Source: CAD feature listing. Evaluate the final solid. Frame: model axes, mm. Face numbers are marked on the shaded views. A direction names the side the tool comes from. Round coordinates to 2 decimals unless told otherwise and drop trailing zeros. Loops run counter-clockwise (first coordinate to the right, second up) from the corner with the lowest first, then second, coordinate; pieces in that order, holes last. Notation, with made-up numbers: (9.5, 0) -> (20.5, 0) arc R21 ccw to (20.5, 39) -> close; hole circle Ø6 at (64, 86.5). An arc over 180 degrees is marked (long way). Put each result on its own line as item: value. Start each with the question number.
1. Cut plane A-A (z = 26). Return the cut outline in (x, y), then the cut area to 3 significant figures.
2. Contact query for flat-ended pins moving along their axis: pin 1 (1.6 mm diameter, centred on x = -38.37, z = 26.15, fed in from +Y); pin 2 (1.5 mm diameter, centred on y = -3.5, z = 33.5, fed in from -X); pin 3 (2 mm diameter, centred on y = -3, z = 30.5, fed in from -X). Output: stop coordinate, or through.
3. Cut plane D-D (x = -34.75). Return the cut outline in (y, z), then the cut area to 3 significant figures.
4. Draft query along Z for the marked faces 1, 2 and 3. Return one class per face: pulls with the +Z half, pulls with the -Z half, needs draft (parallel to the pull), parting line crosses it, or undercut.
5. Cut plane B-B (y = -3.5). State how many separate pieces and enclosed holes the cut face has, then the cut area to 3 significant figures.
6. Material intervals for L1, parallel to Z at x = -30.75, y = -2.5; L2, parallel to Z at x = -38.25, y = -0.5; L3, parallel to X at y = -3.6, z = 28.25, sorted ascending.
7. Set-up query: the marked faces 4, 5 and 6. Return all of +Z, -Z, +X, -X, +Y, -Y with unobstructed straight access to the full face (end or side cutting, diameter ignored); none if empty.
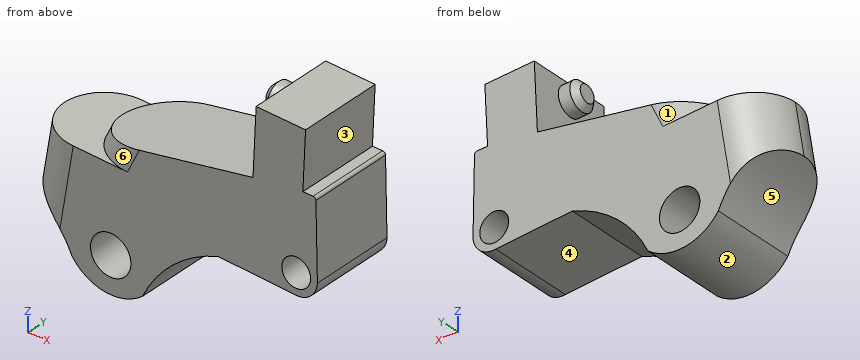
```python
from build123d import *

# Parameters (mm, degrees)
F1_DEPTH = 3.81
F2_D     = 1.778
F3_D     = 1.27
F4_R     = 1.90499
F5_DEPTH = 2.921
F6_R     = 0.636089801
F7_DEPTH = 0.762
F8_SIZE  = 0.254
F9_R     = 0.127


# Not quite as in the source:
# - a fillet or chamfer is up to 0.001 mm smaller than in the source, because OpenCascade refuses the exact size
# - a feature names something its author has since deleted; it is built from what else it names


with BuildPart() as f1:
    # F0 (on Front) → F1 (new body)
    with BuildSketch(Plane.XZ):
        with BuildLine():
            Line((-39.4140869416, 30.484917322), (-39.6941413215, 29.9037330352))
            Line((-39.6941413215, 29.9037330352), (-41.9326054958, 30.025163579))
            Line((-41.9326054958, 30.025163579), (-42.315851897, 27.6998355985))
            ThreePointArc((-42.315851897, 27.6998355985), (-40.9839410359, 26.7856748681), (-40.0724932551, 25.4519060254))
            ThreePointArc((-40.0724932551, 25.4519060254), (-38.6103077884, 24.5752589314), (-36.9695164263, 25.0381845981))
            ThreePointArc((-36.9695164263, 25.0381845981), (-35.6119860231, 26.8367061404), (-33.6415685093, 27.929877378))
            Line((-33.6415685093, 27.929877378), (-30.2701074994, 27.6978733483))
            ThreePointArc((-30.2701074994, 27.6978733483), (-29.5830798604, 27.8997588647), (-29.2723267028, 28.5448923498))
            Line((-29.2723267028, 28.5448923498), (-29.339633882, 31.9740138948))
            Line((-29.339633882, 31.9740138948), (-29.925275594, 31.9827347994))
            Line((-29.925275594, 31.9827347994), (-29.9314986914, 31.6059216857))
            Line((-29.9314986914, 31.6059216857), (-32.1076634707, 31.7085161805))
            Line((-32.1076634707, 31.7085161805), (-39.4140869416, 30.484917322))
        make_face()
    extrude(amount=F1_DEPTH)

    # F2 (through all)
    with Locations(Plane(origin=(0, 0, 0), x_dir=(1, 0, 0), z_dir=(0, 1, 0))):
        with Locations((-38.3695736527, -26.1525325477)):
            Hole(F2_D / 2)

    # F3 (through all)
    with Locations(Plane(origin=(0, 0, 0), x_dir=(1, 0, 0), z_dir=(0, 1, 0))):
        with Locations((-30.2061401308, -28.6094471812)):
            Hole(F3_D / 2)

    # F4 (radius 1.905 in the source; OpenCascade refuses exactly that, so slightly less here)
    f4_edges = [f1.edges().sort_by_distance(p)[0] for p in [
        (-42.124229, -3.81, 28.8625),
        (-42.124229, 0, 28.8625),
        (-39.554114, -3.81, 30.194325),
        (-39.554114, 0, 30.194325),
    ]]
    fillet(f4_edges, radius=F4_R)

    # F5 (add): a face of the model
    f5_faces = [f1.faces().sort_by_distance(p)[0] for p in [
        (-31.0195810811, -1.905, 31.6572189331),
    ]]
    extrude(f5_faces, amount=F5_DEPTH)

    # F6 (on face) → F7 (join)
    with BuildSketch(Plane(origin=(-33.5280299441, 0, 1.5806667432), x_dir=(0, -1, 0), z_dir=(-0.9988905408, 0, 0.0470923302))):
        with Locations((1.905, 32.3275662959)):
            Circle(F6_R)
    extrude(amount=F7_DEPTH)

    # F8
    f8_edges = [f1.edges().sort_by_distance(p)[0] for p in [
        (-32.766804, -1.26891, 33.908251),
    ]]
    chamfer(f8_edges, length=F8_SIZE)

    # F9
    f9_edges = [f1.edges().sort_by_distance(p)[0] for p in [
        (-29.339634, -1.905, 31.974014),
    ]]
    fillet(f9_edges, radius=F9_R)


solid = f1.part
```
Solution:
1. outline: (-40.36, -3.81) -> (-39.25, -3.81) -> (-39.25, 0) -> (-40.36, 0) -> close; (-37.49, -3.81) -> (-36.39, -3.81) -> (-36.39, 0) -> (-37.49, 0) -> close
1. area: 8.45 mm^2
2. pin 1: passes through
2. pin 2: stops at x = -32.06
2. pin 3: stops at x = -41.93
3. outline: (-3.81, 27.45) -> (0, 27.45) -> (0, 31.27) -> (-3.81, 31.27) -> close
3. area: 14.5 mm^2
4. face 1: pulls with the +Z half
4. face 2: pulls with the -Z half
4. face 3: undercut
5. separate pieces: 1
5. enclosed holes: 2
5. area: 55.2 mm^2
6. L1: z = 27.73 to 28.28, 28.94 to 34.57
6. L2: z = 24.56 to 25.27, 27.03 to 30.68
6. L3: x = -41.18 to -30.73, -29.68 to -29.33
7. face 4: -Z, +Y, -Y
7. face 5: -Z, -X, +Y, -Y
7. face 6: +Z, -Y
